The listing builds one solid part. Answer for the finished solid, in the listing's coordinates (mm). Face numbers are marked on the shaded views. Coordinates: 2 decimals unless noted, no trailing zeros. Order: outer loops, then holes, each group sorted by start corner. A loop starts at its lowest first (then second) coordinate and runs counter-clockwise, first axis right, second up. Notation, with made-up numbers: (62, 72.25) -> (121, 72.25) arc R27 ccw to (121, 90.25) -> close; hole circle Ø4 at (63.5, 14.5). An arc over 180 degrees is marked (long way). One line per question, with ' | ' between items.
Autodesk Inventor part; units mm, degrees
ref_plane "Work Plane1" through (20, 0, 0) normal (1, 0, 0) x (0, 1, 0)
ref_plane "XZ Plane" through (0, 0, 0) normal (0, 1, 0) x (-1, 0, 0)
ref_plane "XY Plane" through (0, 0, 0) normal (0, 0, 1) x (1, 0, 0)
sketch "Sketch1" plane through (0, 0, 0) normal (0, 0, 1) x (1, 0, 0)
  line L0 (0, 0) -> (0, 44.0101) construction
  line L1 (33.5, 0) -> (33.5, -20.5)
  line L2 (33.5, -20.5) -> (-33.5, -20.5)
  line L3 (-33.5, -20.5) -> (-33.5, 0)
  arc A0 (-6.975, 0) -> (6.975, 0) centre (0, 0) ccw
  line L4 (-33.5, 0) -> (-6.975, 0)
  line L5 (6.975, 0) -> (33.5, 0)
  dimension "d0" = 67
  dimension "d1" = 20.5
  dimension "d2" = 6.975
extrude "Extrusion1" add sketch "Sketch1" along normal mid plane 129
ref_plane "Work Plane1" through (20, 0, 0) normal (1, 0, 0) x (0, 1, 0)
sketch "Sketch2" plane through (20, 0, 0) normal (1, 0, 0) x (0, 1, 0)
  line L0 (-6.975, 64.5) -> (0, 64.5)
  line L1 (0, 64.5) -> (8, 64.5)
  line L2 (7.0278, 62) -> (2, 62)
  line L3 (10, 62.5) -> (10, 59)
  line L4 (8, 57) -> (5, 57)
  arc A0 (7.0278, 58.9998) -> (5, 57) centre (7, 57) ccw
  line L5 (7.0278, 62) -> (7.0278, 58.9998)
  line L6 (0, -64.5) -> (0, 64.5)
  arc A1 (2, 62) -> (0, 60) centre (2, 60) ccw
  arc A2 (10, 62.5) -> (8, 64.5) centre (8, 62.5) ccw
  arc A3 (8, 57) -> (10, 59) centre (8, 59) ccw
  point P0 (0, 0)
  point P1 (10, 64.5)
  point P2 (0.0278, 62)
  point P3 (10, 57)
  dimension "d6" = 10
  dimension "d8" = 2.5
  dimension "d12" = 7
  dimension "d13" = 7.5
  dimension "d14" = 5
  dimension "d15" = 2
  dimension "d16" = 2
  dimension "d19" = 2
extrude "Extrusion2" add sketch "Sketch2" along normal mid plane 5
mirror "Mirror1" about plane through (0, 0, 0) normal (1, 0, 0) of "Extrusion2"
properties part number "Laser_Pen_Housing"
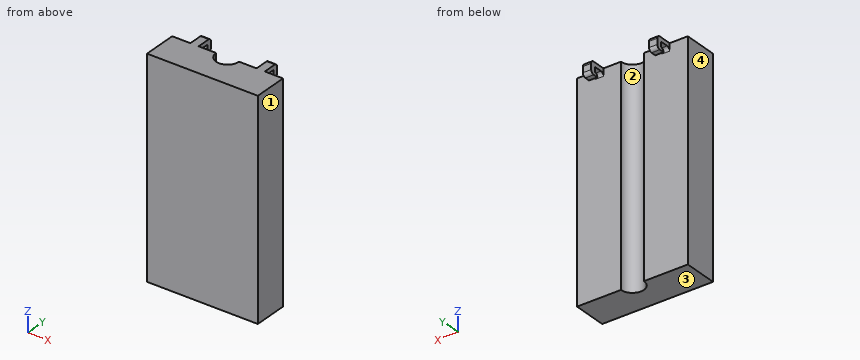
Item 1: Section A-A, the plane y = -2 is taken. Give the vertices of the cut face in (x, z), plus the area to 3 significant figures.
Computed values:
outline: (-33.5, -64.5) -> (-6.68, -64.5) -> (-6.68, 64.5) -> (-33.5, 64.5) -> close; (6.68, -64.5) -> (33.5, -64.5) -> (33.5, 64.5) -> (6.68, 64.5) -> close | area: 6,920 mm^2
Item 2: Section D-D, the plane x = 0 is taken. Give the vertices of the cut face in (y, z) (3 decimals), plus the area to 3 significant figures.
Computed values:
outline: (-20.5, -64.5) -> (-6.975, -64.5) -> (-6.975, 64.5) -> (-20.5, 64.5) -> close | area: 1,740 mm^2
Item 3: Section B-B, the plane x = 11 is taken. Give the vertices of the cut face in (y, z).
Computed values:
outline: (-20.5, -64.5) -> (0, -64.5) -> (0, 64.5) -> (-20.5, 64.5) -> close
Item 4: Find the intervals of material crossed by L1, parallel to Y at x = -30, z = 14.5; L2, parallel to X at y = -4.5, z = -16; L3, parallel to X at y = -1, z = 56, in increasing order.
Computed values:
L1: y = -20.5 to 0 | L2: x = -33.5 to -5.33, 5.33 to 33.5 | L3: x = -33.5 to -6.9, 6.9 to 33.5
Item 5: Each of these flat-tipped pins is pushed along its axis until it touches: pin 1 Ø3.5 at (x, y) = (20.5, 6.5) entering from -Z; pin 2 Ø10 at (y, z) = (1.5, -7.5) entering from -X; pin 3 Ø4 at (y, z) = (6.5, 59) entering from +X; pin 4 Ø5 at (x, z) = (19, 43.5) entering from +Y. Where does it stop, or does it pass through?
Computed values:
pin 1: stops at z = 57 | pin 2: stops at x = -33.5 | pin 3: stops at x = 22.5 | pin 4: stops at y = 0
Item 6: Section C-C, the plane z = 41.5 is taken. Give the vertices of the cut face in (x, y) (3 decimals).
Computed values:
outline: (-33.5, -20.5) -> (33.5, -20.5) -> (33.5, 0) -> (6.975, 0) arc R6.975 cw to (-6.975, 0) -> (-33.5, 0) -> close
Item 7: Determine the mould class of the marked faces 1, 2, 3 and 4 for opening direction X: pulls with the +X half, pulls with the -X half, needs draft (parallel to the pull), parting line crosses it, or undercut.
Computed values:
face 1: pulls with the +X half | face 2: undercut | face 3: needs draft | face 4: pulls with the -X half
